Geometry check sheet. Reference: drawing and pictorial views, mm from the part's lowest x, y, z. Give positions to 0.01 mm unless a question says otherwise; leave off trailing zeros. Order: outer loops, then holes, each group sorted by start corner. A loop starts at its lowest first (then second) coordinate and runs counter-clockwise, first axis right, second up. Notation, with made-up numbers: (69, 16) -> (108, 16) arc R27 ccw to (108, 39) -> close; hole circle Ø9 at (-16, 63.25). An arc over 180 degrees is marked (long way). Write each question's results on one line, items separated by ' | '. Start each with the question number.
1. Cross-section at A-A, the plane y = 180. Enter the section's corners in (x, z), then the cut area to 3 significant figures.
2. Material ranges on L1, parallel to Y at x = 180, z = 2.5; L2, parallel to X at y = 15.5, z = 1.5, recorded low to high. Write a range as from..to.
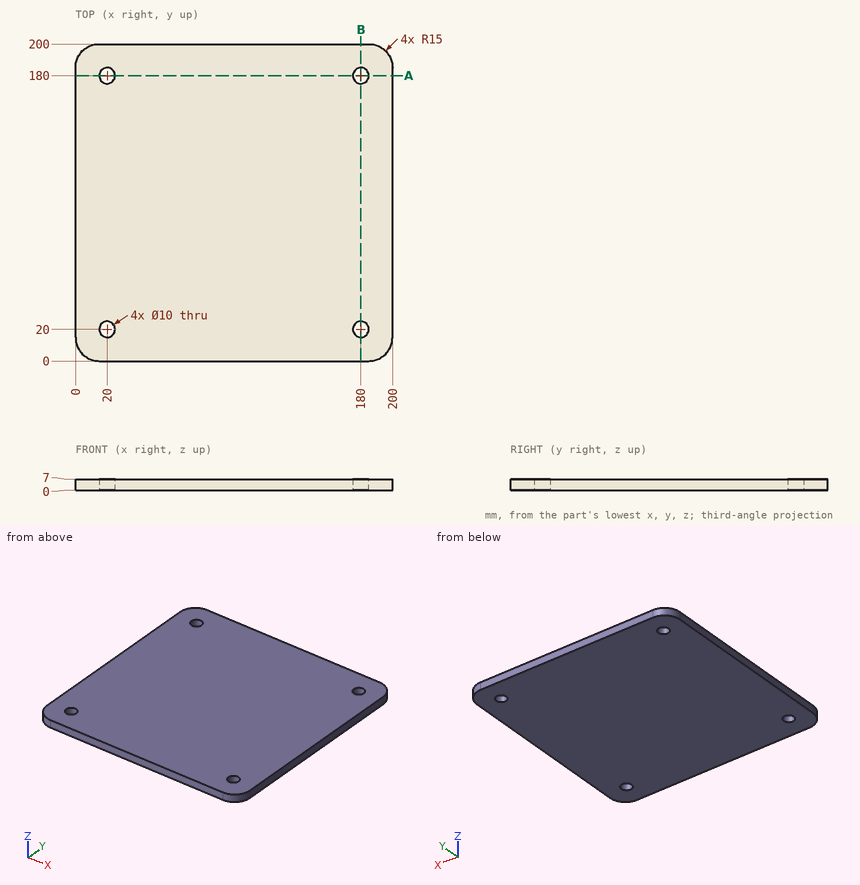
Results below:
1) outline: (0, 0) -> (15, 0) -> (15, 7) -> (0, 7) -> close; (25, 0) -> (175, 0) -> (175, 7) -> (25, 7) -> close; (185, 0) -> (200, 0) -> (200, 7) -> (185, 7) -> close | area: 1,260 mm²
2) L1: y = 0..15, 25..175, 185..200 | L2: x = 0..17.82, 22.18..177.82, 182.18..200
